Autodesk Inventor part; units mm, degrees
ref_plane "YZ Plane" through (0, 0, 0) normal (1, 0, 0) x (0, 1, 0)
ref_plane "XZ Plane" through (0, 0, 0) normal (0, 1, 0) x (-1, 0, 0)
ref_plane "XY Plane" through (0, 0, 0) normal (0, 0, 1) x (1, 0, 0)
sketch "Sketch1" plane through (0, 0, 0) normal (0, 0, 1) x (1, 0, 0)
  line L0 (43.3013, -75) -> (-43.3013, -75)
  line L1 (-43.3013, -75) -> (-86.6025, 0)
  line L2 (-86.6025, 0) -> (-43.3013, 75)
  line L3 (-43.3013, 75) -> (43.3013, 75)
  line L4 (43.3013, 75) -> (86.6025, 0)
  line L5 (86.6025, 0) -> (43.3013, -75)
  point P0 (0, 0)
  point P1 (0, 0)
  dimension "d0" = 150
extrude "Extrusion1" add sketch "Sketch1" along normal blind 2
sketch "Sketch5" plane through (0, 0, 2) normal (0, 0, 1) x (1, 0, 0)
  line L0 (-43.3013, -75) -> (43.3013, -75)
  line L1 (43.3013, -75) -> (86.6025, 0)
  line L2 (86.6025, 0) -> (43.3013, 75)
  line L3 (43.3013, 75) -> (-43.3013, 75)
  line L4 (-43.3013, 75) -> (-86.6025, 0)
  line L5 (-86.6025, 0) -> (-43.3013, -75)
  line L6 (-84.2931, 0) -> (-42.1466, 73)
  line L7 (-42.1466, 73) -> (42.1466, 73)
  line L8 (42.1466, 73) -> (84.2931, 0)
  line L9 (84.2931, 0) -> (42.1466, -73)
  line L10 (42.1466, -73) -> (-42.1466, -73)
  line L11 (-42.1466, -73) -> (-84.2931, 0)
  line L12 (-81.9837, 0) -> (-40.9919, 71)
  line L13 (-40.9919, 71) -> (40.9919, 71)
  line L14 (40.9919, 71) -> (81.9837, 0)
  line L15 (81.9837, 0) -> (40.9919, -71)
  line L16 (40.9919, -71) -> (-40.9919, -71)
  line L17 (-40.9919, -71) -> (-81.9837, 0)
  point P0 (0, 0)
  dimension "d15" = 2
  dimension "d16" = 2
extrude "Extrusion5" add sketch "Sketch5" along normal blind 10 contours L6 L7 L8 L9 L10 L11
sketch "Sketch7" plane through (0, 0, 2) normal (0, 0, 1) x (1, 0, 0)
  line L0 (40.9919, 71) -> (-40.9919, 71)
  line L1 (-40.9919, 71) -> (-81.9837, 0)
  line L2 (-81.9837, 0) -> (-40.9919, -71)
  line L3 (-40.9919, -71) -> (40.9919, -71)
  line L4 (40.9919, -71) -> (81.9837, 0)
  line L5 (81.9837, 0) -> (40.9919, 71)
  line L6 (-38.6825, -67) -> (-77.3649, 0)
  line L7 (-77.3649, 0) -> (-38.6825, 67)
  line L8 (-38.6825, 67) -> (38.6825, 67)
  line L9 (38.6825, 67) -> (77.3649, 0)
  line L10 (77.3649, 0) -> (38.6825, -67)
  line L11 (38.6825, -67) -> (-38.6825, -67)
  point P0 (0, 0)
  dimension "d19" = 4
extrude "Extrusion6" cut sketch "Sketch7" against normal blind 7 contours L6 L7 L8 L9 L10 L11
fillet "Fillet1" radius 10 6 edges at (43.3013, 75, 1) (86.6025, 0, 1) (43.3013, -75, 1) (-43.3013, -75, 1) (-86.6025, 0, 1) (-43.3013, 75, 1)
fillet "Fillet1" radius 4 12 edges at (42.1466, -73, 7) (-40.9919, -71, 7) (-84.2931, 0, 7) (-42.1466, 73, 7) (42.1466, 73, 7) (84.2931, 0, 7) (40.9919, -71, 7) (81.9837, 0, 7) (-40.9919, 71, 7) (40.9919, 71, 7) (-42.1466, -73, 7) (-81.9837, 0, 7)
fillet "Fillet2" radius 10 6 edges at (38.6825, -67, 1) (77.3649, 0, 1) (38.6825, 67, 1) (-38.6825, 67, 1) (-77.3649, 0, 1) (-38.6825, -67, 1)
properties part number "Cover v1"
For this review, take the finished solid that the model builds, in its own axes (mm). A direction names the side the tool comes from. Coordinates: 2 decimals unless noted, no trailing zeros. Loops run counter-clockwise (first coordinate to the right, second up) from the corner with the lowest first, then second, coordinate; pieces in that order, holes last.
1. Add section C-C, the plane y = 40. Give the boundary of the cut face in (x, z).
2. Add section B-B, the plane z = 8. Give the boundary of the cut face in (x, y).
3. For line 1 (Y direction, x = -25, z = 3.75); line 2 (Y direction, x = 13.5, z = 1.25); line 3 (X direction, y = 14.5, z = 1.25), list the stretches that pass through material, from the lowest coordinate up.
4. Mouldability with a two-part tool opening along X and no side actions: class faces 5 (the cylindrical face through (42.591, 73.623, 1.014)), 6 (the cylindrical face through (-42.591, -73.623, 1.014)), 7 (the cylindrical face through (-37.972, 65.623, 0.986)) as +X half, -X half, draft (parallel to the pull), parting line (faces both ways), or undercut.
5. Add section A-A, the plane x = 24. Give the boundary of the cut face in (y, z), then the cut area to 3 significant figures.
6. For faces 1 (the flat face through (-1, 71, 7)), 2 (the cylindrical face through (-83.674, 0.029, 7.07)), 3 (the cylindrical face through (41.81, -72.48, 7.07)), 4 (the cylindrical face through (-37.845, -65.697, 0.986)), list the 3-axis set-ups (+Z, -Z, +X, -X, +Y, -Y) from which the entire face can be reached by the end or side of a thin tool; tool diameter is ignored.
7. Insertion check: P1, Ø3, axis at x = -8.5, z = 6, coming from the +Y side; P2, Ø3, axis at y = 27.5, z = 5, coming from the -X side; P3, Ø6, axis at y = -59, z = 3, coming from the -X side. Each pin has a flat end and moves straight along its axis. Give the tip position at first contact, or say it passes through.
Result:
1. outline: (-63.51, 0) - (-54.27, 0) - (-54.27, 2) - (-58.89, 2) - (-58.89, 12) - (-61.2, 12) - (-61.2, 2) - (-63.51, 2) - close; (54.27, 0) - (63.51, 0) - (63.51, 2) - (61.2, 2) - (61.2, 12) - (58.89, 12) - (58.89, 2) - (54.27, 2) - close
2. outline: (-83.14, -2) - (-43.3, -71) arc R4 ccw to (-39.84, -73) - (39.84, -73) arc R4 ccw to (43.3, -71) - (83.14, -2) arc R4 ccw to (83.14, 2) - (43.3, 71) arc R4 ccw to (39.84, 73) - (-39.84, 73) arc R4 ccw to (-43.3, 71) - (-83.14, 2) arc R4 ccw to start; hole (-80.83, -2) - (-42.15, -69) arc R4 ccw to (-38.68, -71) - (38.68, -71) arc R4 ccw to (42.15, -69) - (80.83, -2) arc R4 ccw to (80.83, 2) - (42.15, 69) arc R4 ccw to (38.68, 71) - (-38.68, 71) arc R4 ccw to (-42.15, 69) - (-80.83, 2) arc R4 ccw to start
3. line 1: y = -73 to -71, 71 to 73
3. line 2: y = -75 to -67, 67 to 75
3. line 3: x = -78.23 to -68.99, 68.99 to 78.23
4. face 5: +X half
4. face 6: -X half
4. face 7: undercut
5. outline: (-75, 0) - (-67, 0) - (-67, 2) - (-71, 2) - (-71, 12) - (-73, 12) - (-73, 2) - (-75, 2) - close; (67, 0) - (75, 0) - (75, 2) - (73, 2) - (73, 12) - (71, 12) - (71, 2) - (67, 2) - close
5. area: 72.0 mm2
6. face 1: +Z
6. face 2: +Z, -X
6. face 3: +Z, +X, -Y
6. face 4: +Z, -Z
7. P1: stops at y = 73
7. P2: stops at x = -69.28
7. P3: stops at x = -54.17
